Can you work these out from the model? Positions are in its coordinate system, mm. Round coordinates to 2 decimals unless told otherwise and drop trailing zeros. Loops run counter-clockwise (first coordinate to the right, second up) from the corner with the lowest first, then second, coordinate; pieces in that order, holes last. Notation, with made-up numbers: (43.25, 56) -> (90.25, 56) arc R34 cw to (90.25, 88) -> close; hole circle Ø1 at (43, 4.5). An arc over 180 degrees is marked (long way). Answer as a JSON object with one key per item and string values.
Autodesk Inventor part; units mm, degrees
ref_plane "YZ Plane" through (0, 0, 0) normal (1, 0, 0) x (0, 1, 0)
ref_plane "XZ Plane" through (0, 0, 0) normal (0, 1, 0) x (-1, 0, 0)
ref_plane "XY Plane" through (0, 0, 0) normal (0, 0, 1) x (1, 0, 0)
sketch "スケッチ1" plane through (0, 0, 0) normal (1, 0, 0) x (0, 1, 0)
  circle A0 centre (0, 0) radius 13
  circle A1 centre (0, 0) radius 4.25
  circle A2 centre (0, 0) radius 6 construction
  circle A3 centre (6, 0) radius 1
  circle A4 centre (3, 5.1962) radius 1
  circle A5 centre (-3, 5.1962) radius 1
  circle A6 centre (-6, 0) radius 1
  circle A7 centre (-3, -5.1962) radius 1
  circle A8 centre (3, -5.1962) radius 1
  line L0 (0, 13) -> (-44.9356, 13)
  line L1 (-44.9356, 13) -> (-44.9356, -13)
  line L2 (-44.9356, -13) -> (0, -13)
  line L3 (0, -13) -> (0, 13)
  line L4 (-20, 6.3185) -> (-25.1764, -13)
  line L5 (-25.1764, -13) -> (-92.7912, 5.1173)
  line L6 (-92.7912, 5.1173) -> (-87.6148, 24.4358)
  line L7 (-87.6148, 24.4358) -> (-20, 6.3185)
  line L8 (-68.643, 19.3524) -> (-90.5498, 13.4825)
  line L9 (-87.9616, 3.8232) -> (-90.5498, 13.4825)
  circle A9 centre (-72.0415, 13.3611) radius 2.5
  circle A10 centre (-60.509, 10.271) radius 2.5
  circle A11 centre (-79.5332, 8.4667) radius 2.5
  circle A12 centre (-68.0007, 5.3766) radius 2.5
  circle A13 centre (-56.4682, 2.2864) radius 2.5
  line L10 (-72.0415, 13.3611) -> (-60.509, 10.271) construction
  line L11 (-79.5332, 8.4667) -> (-56.4682, 2.2864) construction
  line L12 (-72.0415, 13.3611) -> (-72.6885, 10.9463) construction
  line L13 (-79.5332, 8.4667) -> (-80.1803, 6.0519) construction
  line L14 (-68.0007, 5.3766) -> (-68.6477, 2.9618) construction
  line L15 (-79.5332, 8.4667) -> (-89.9539, 11.2589) construction
  line L16 (-56.4682, 2.2864) -> (-44.9356, -0.8037) construction
  line L17 (-56.4682, 2.2864) -> (-57.1152, -0.1284)
  point P0 (-3.3656, 12.5568)
  point P1 (-44.9356, -7.7055)
  dimension "d2" = 26
  dimension "d4" = 12
  dimension "d27" = 5
  dimension "d29" = 5
  dimension "d30" = 5
  dimension "d31" = 5
  dimension "d3" = 8.5
  dimension "d5" = 2
  dimension "d8" = 360
  dimension "d12" = 15
  dimension "d13" = 20
  dimension "d14" = 70
  dimension "d15" = 20
  dimension "d18" = 10
  dimension "d19" = 30
  dimension "d28" = 5
  dimension "d32" = 11.9393
  dimension "d33" = 11.9393
  dimension "d34" = 11.9393
  dimension "d35" = 5.9697
  dimension "d36" = 6.6667
  dimension "d37" = 6.6667
  dimension "d38" = 6.6667
  dimension "d39" = 11.9393
  dimension "d40" = 11.9393
extrude "押し出し1" add sketch "スケッチ1" along normal blind 1.5 contours L1 L5 L9 L8 L7 | A9 | A10 | A11 | A12 | A13
fillet "フィレット1" radius 5 5 edges at (0.75, -68.643, 19.3524) (0.75, -90.5498, 13.4825) (0.75, -87.9616, 3.8232) (0.75, -44.9356, -7.7055) (0.75, -44.9356, 13)
sketch "スケッチ3" plane through (1.5, 0, 0) normal (1, 0, 0) x (0, 0, -1)
  point P0 (0, 0)
sketch "スケッチ4" plane through (1.5, 0, 0) normal (1, 0, 0) x (0, 0, -1)
  circle A0 centre (-9.947, -84.426) radius 0.8
  circle A1 centre (-11.2411, -79.5964) radius 0.8
  circle A2 centre (-14.176, -68.643) radius 0.8
  circle A3 centre (-9.1634, -49.9356) radius 0.8
  circle A4 centre (1.1894, -49.9356) radius 0.8
  circle A5 centre (-3.8232, -68.643) radius 0.8
  arc A6 (-19.0056, -67.3489) -> (-19.0056, -69.9371) centre (-14.176, -68.643) ccw
  arc A7 (-9.1634, -44.9356) -> (-13.993, -48.6415) centre (-9.1634, -49.9356) ccw
  arc A8 (6.019, -51.2297) -> (1.1894, -44.9356) centre (1.1894, -49.9356) ccw
  line L0 (-3.8232, -68.643) -> (1.1894, -49.9356) construction
  line L1 (-3.0761, -85.1732) -> (6.019, -51.2297)
  point P0 (0, 0)
  dimension "d43" = 1.6
  dimension "d44" = 1.6
  dimension "d45" = 1.6
  dimension "d46" = 1.6
extrude "押し出し2" cut sketch "スケッチ4" against normal through all
equation "\"d32\" = d40"
equation "\"d33\" = d32"
equation "\"d34\" = d33"
equation "\"d35\" = 0.5 * d33"
equation "\"d36\" = d38"
equation "\"d37\" = d38"
equation "\"d39\" = d40"
properties part number "hand" material "アルミニウム 6061"
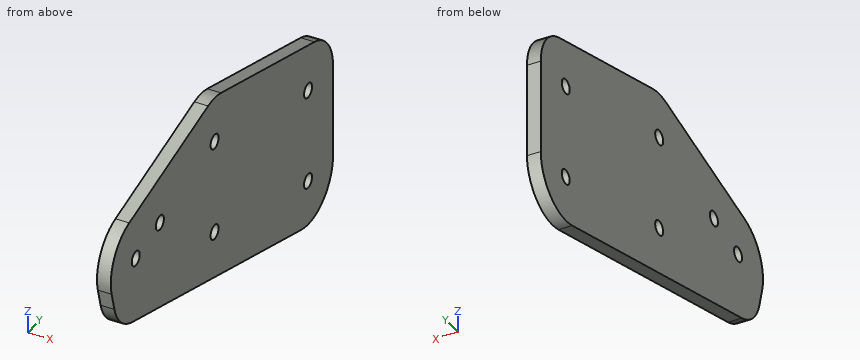
Q1. I want a section at D-D, the plane z = 3.75. Write out the boundary of the cut face in (x, y), then the cut area to 3 significant figures.
Determined:
{"outline": "(0, -86.66) -> (1.5, -86.66) -> (1.5, -69.44) -> (0, -69.44) -> close; (0, -67.85) -> (1.5, -67.85) -> (1.5, -44.94) -> (0, -44.94) -> close", "area": "60.2 mm²"}
Q2. I'm going to push a flat-ended pin straight in: pin 1 (1.3 mm diameter, centred on y = -49.94, z = 9.16, fed in from -X). Where does the tip first touch, or does it pass through?
Determined:
{"pin 1": "through"}
Q3. If I drill on L1, parallel to Y at x = 0.45, z = 9.75; L2, parallel to Y at x = 0.95, z = 10; L3, parallel to Y at x = 1.2, z = 4, over which ranges is the centre line in solid material (lowest first)? Write a range as [from, to].
Determined:
{"L1": "[-89.42, -85.2], [-83.65, -50.48], [-49.39, -44.97]", "L2": "[-89.43, -85.22], [-83.63, -45.01]", "L3": "[-87, -69.42], [-67.86, -44.94]"}
Q4. I want a section at B-B, the plane x = 0.25. Write out the boundary of the cut face in (y, z), then the cut area to 3 significant figures.
Determined:
{"outline": "(-89.26, 8.65) -> (-88.71, 6.61) arc R5 ccw to (-85.17, 3.08) -> (-51.23, -6.02) arc R5 ccw to (-44.94, -1.19) -> (-44.94, 9.16) arc R5 ccw to (-48.64, 13.99) -> (-67.35, 19.01) arc R5 ccw to (-69.94, 19.01) -> (-85.72, 14.78) arc R5 ccw to start; hole circle Ø1.6 at (-84.43, 9.95); hole circle Ø1.6 at (-79.6, 11.24); hole circle Ø1.6 at (-68.64, 3.82); hole circle Ø1.6 at (-68.64, 14.18); hole circle Ø1.6 at (-49.94, -1.19); hole circle Ø1.6 at (-49.94, 9.16)", "area": "773 mm²"}
Q5. I want a section at C-C, the plane y = -54. Write out the boundary of the cut face in (x, z).
Determined:
{"outline": "(0, -5.28) -> (1.5, -5.28) -> (1.5, 15.43) -> (0, 15.43) -> close"}
Q6. I want a section at A-A, the plane z = 11.25. Write out the boundary of the cut face in (x, y).
Determined:
{"outline": "(0, -89.25) -> (1.5, -89.25) -> (1.5, -80.4) -> (0, -80.4) -> close; (0, -78.8) -> (1.5, -78.8) -> (1.5, -45.39) -> (0, -45.39) -> close"}
